Can you work these out from the drawing? Everything is in mm from the part's minimum corner. Round coordinates to 2 decimals unless told otherwise and drop trailing zeros. Loops run counter-clockwise (first coordinate to the right, second up) from the corner with the lowest first, then second, coordinate; pieces in that order, holes last. Notation, with made-up numbers: M 84.25,63 L 107.25,63 A14 ccw 107.25,83 Z; hole C 8.25,85.5 d10. An arc over 180 degrees is marked long. Return JSON: item names as keys, results as strings. Group by question number.
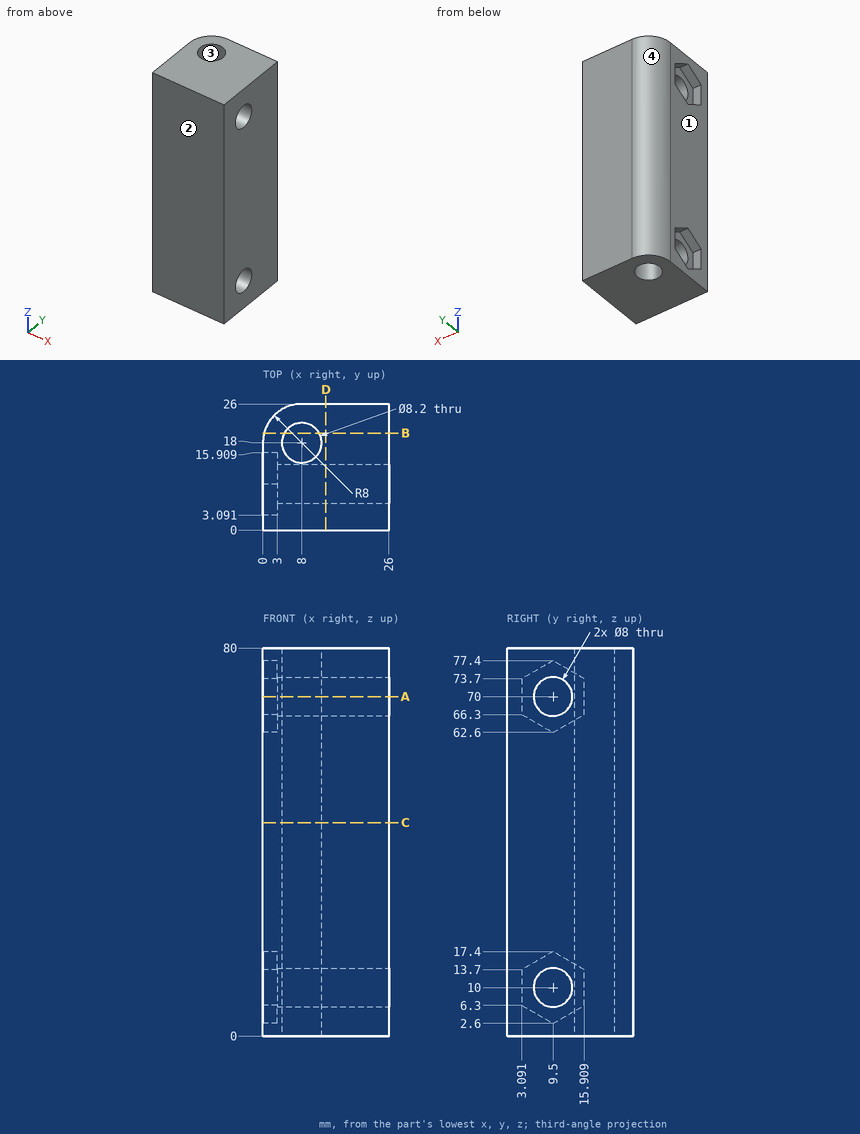
1. If we section it at B-B, the plane y = 20: Please give me the cut outline in (x, z).
2. I'm going to push flat-ended pins straight in: pin 1 Ø6.5 at (y, z) = (9.5, 70) entering from +X; pin 2 Ø1.5 at (x, z) = (1, 69.5) entering from +Y (1 decimal); pin 3 Ø2.5 at (x, z) = (1.5, 11) entering from +Y (1 decimal). Where does each tip first touch, or does it pass through?
3. I need wall thicknesses on probe 1 along Z at (x, y) = (1.75, 14); probe 2 along Z at (x, y) = (16.75, 8.25); probe 3 along Y at (x, z) = (4.5, 75.5) (1 decimal). Which ranges of each line are inside material? Lowest first, please.
4. If we section it at D-D, the plane x = 13: Please give me the cut outline in (y, z), then the cut area to 3 significant figures.
5. If we section it at C-C, the plane z = 44: Please give me the cut outline in (x, y).
6. We'd pull the mould along Y, two halves only. Please class the marked faces 1, 2, 3 and 4: +Y half, -Y half, draft (parallel to the pull), parting line (faces both ways), or undercut.
7. If we section it at A-A, the plane z = 70: Please give me the cut outline in (x, y).
Geometry results:
{
 "1": {"outline": "M 0.25,0 L 4.42,0 L 4.42,80 L 0.25,80 Z; M 11.58,0 L 26,0 L 26,80 L 11.58,80 Z"},
 "2": {"pin 1": "through", "pin 2": "y = 23", "pin 3": "y = 24"},
 "3": {"probe 1": "0 to 5.2, 14.8 to 65.2, 74.8 to 80", "probe 2": "0 to 6.2, 13.8 to 66.2, 73.8 to 80", "probe 3": "0 to 15.9, 20.1 to 25.2"},
 "4": {"outline": "M 0,0 L 26,0 L 26,80 L 0,80 Z; hole C 9.5,10 d8; hole C 9.5,70 d8", "area": "1,980 mm^2"},
 "5": {"outline": "M 0,0 L 26,0 L 26,26 L 8,26 A8 ccw 0,18 Z; hole C 8,18 d8.2"},
 "6": {"face 1": "draft", "face 2": "-Y half", "face 3": "undercut", "face 4": "+Y half"},
 "7": {"outline": "M 0,0 L 26,0 L 26,5.5 L 3,5.5 L 3,3.09 L 0,3.09 Z; M 0,15.91 L 3,15.91 L 3,13.5 L 26,13.5 L 26,26 L 8,26 A8 ccw 0,18 Z; hole C 8,18 d8.2"}
}
